Design review of the part built by this model. Coordinates are the model's own, in mm. Coordinates: 2 decimals unless noted, no trailing zeros. Write each loop counter-clockwise with the first axis right and the second up, starting at its lowest first coordinate (ties: lowest second). Pieces come first, ordered by that corner, then holes. Notation, with made-up numbers: M -13,-11 L 30,-11 A28 cw 30,24 Z; hole C 20.25,56.5 d7. An arc over 180 degrees is marked long. One line per question, with ' | ' between items.
from build123d import *

# Parameters (mm, degrees)
PAD001_DEPTH = 0.3
FILLET004_R  = 0.1
FILLET005_R  = 0.1


with BuildPart() as part:
    # Sketch002 → Pad001 (new body)
    with BuildSketch(Plane.XY):
        with BuildLine():
            Line((0, 12.098547), (7, 17))
            Line((7, 17), (0.3, 17))
            ThreePointArc((0.3, 17), (0.087868, 16.912132), (0, 16.7))
            Line((0, 12.098547), (0, 16.7))
        make_face()
    extrude(amount=PAD001_DEPTH)

    # Fillet004
    fillet004_edges = [part.edges().sort_by_distance(p)[0] for p in [
        (0, 14.399274, 0.3),
        (0.087868, 16.912132, 0.3),
        (3.65, 17, 0.3),
    ]]
    fillet(fillet004_edges, radius=FILLET004_R)

    # Fillet005
    fillet005_edges = [part.edges().sort_by_distance(p)[0] for p in [
        (0, 14.399274, 0),
        (0.087868, 16.912132, 0),
        (3.65, 17, 0),
    ]]
    fillet(fillet005_edges, radius=FILLET005_R)


solid = part.part
1. Take a section at C-C (z = 0.15). Write out the cut boundary in (x, y), then the cut area to 3 significant figures.
Answer sheet:
outline: M 0,12.1 L 7,17 L 0.3,17 A0.3 ccw 0,16.7 Z | area: 17.1 mm^2
2. Take a section at A-A (x = 1.25). Write out the cut boundary in (y, z).
Answer sheet:
outline: M 12.97,0 L 16.9,0 A0.1 ccw 17,0.1 L 17,0.2 A0.1 ccw 16.9,0.3 L 12.97,0.3 Z
3. To check wall thickness, follow line 1 along Y through (x, z) = (5, 0.1); line 2 along Y through (x, z) = (2, 0.15); line 3 along X through (y, z) = (16.7, 0.1). State the ranges of each line that lie inside material, in increasing order. Write a range as [from, to].
Answer sheet:
line 1: [15.6, 17] | line 2: [13.5, 17] | line 3: [0, 6.57]
4. Take a section at B-B (y = 13.35). Write out the cut boundary in (x, z), then the cut area to 3 significant figures.
Answer sheet:
outline: M 0,0.1 A0.1 ccw 0.1,0 L 1.79,0 L 1.79,0.3 L 0.1,0.3 A0.1 ccw 0,0.2 Z | area: 0.532 mm^2
